The listing builds one solid part. Answer for the finished solid, in the listing's coordinates (mm). Give positions to 0.01 mm unless a question says otherwise; leave off trailing zeros. Write each loop counter-clockwise with the first axis right and the second up, starting at its lowest first coordinate (ties: lowest second). Pieces come first, ordered by that corner, then holes. Notation, with made-up numbers: (84, -2.75) -> (88, -2.75) arc R19 ccw to (88, 9.25) -> close; hole circle Ø7 at (74.5, 89.25). An arc over 180 degrees is marked (long way). One line per question, with ' | ' between items.
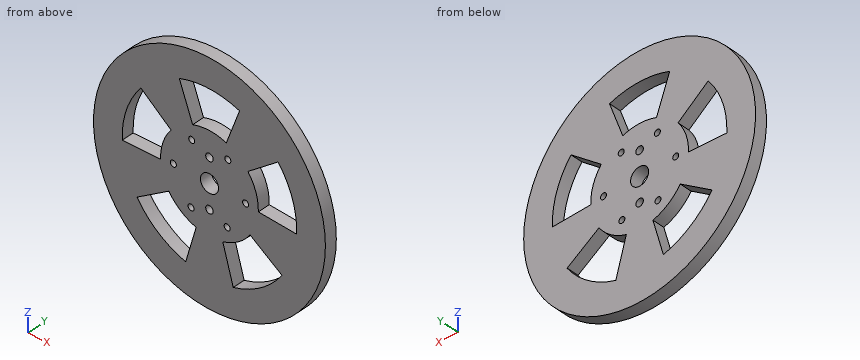
from build123d import *

# Parameters (mm, degrees)
F0_R            = 244.475
F0_R_2          = 6.35
F0_R_3          = 7.9375
F0_R_4          = 19.05
F1_DEPTH        = 25.4
F3_DEPTH        = 25.4
F3_COPIES_COUNT = 5


# Not quite as in the source:
# - a pattern or mirror of a feature is missing from the dataset's text; its kind, count and spacing are read off the source's solid


with BuildPart() as f1:
    # F0 (on Front) → F1 (new body)
    with BuildSketch(Plane.XZ):
        Circle(F0_R)
        with Locations((-38.7905028095, -65.5876275817)):
            Circle(F0_R_2, mode=Mode.SUBTRACT)
        with Locations((37.4053002549, -66.3873746494)):
            Circle(F0_R_2, mode=Mode.SUBTRACT)
        with Locations((0, -50.8)):
            Circle(F0_R_3, mode=Mode.SUBTRACT)
        with Locations((76.1958030644, -0.7997470677)):
            Circle(F0_R_2, mode=Mode.SUBTRACT)
        with Locations((-76.1958030644, 0.7997470677)):
            Circle(F0_R_2, mode=Mode.SUBTRACT)
        with Locations((-37.4053002549, 66.3873746494)):
            Circle(F0_R_2, mode=Mode.SUBTRACT)
        Circle(F0_R_4, mode=Mode.SUBTRACT)
        with Locations((0, 50.8)):
            Circle(F0_R_3, mode=Mode.SUBTRACT)
        with Locations((38.7905028095, 65.5876275817)):
            Circle(F0_R_2, mode=Mode.SUBTRACT)
    extrude(amount=F1_DEPTH)

    # F2 (on Front) → F3 (cut, through all)
    with BuildSketch(Plane.XZ):
        with BuildLine():
            ThreePointArc((-35.5586123208, 96.7233082276), (0, 103.0524782073), (35.5586123208, 96.7233082276))
            Line((35.5586123208, 96.7233082276), (63.5, 172.7269336903))
            ThreePointArc((63.5, 172.7269336903), (0, 184.0294640053), (-63.5, 172.7269336903))
            Line((-63.5, 172.7269336903), (-35.5586123208, 96.7233082276))
        make_face()
    f3 = extrude(amount=F3_DEPTH, mode=Mode.SUBTRACT)

    # F3_copies: F3 ×5 about axis
    f3_copies_axis = Axis((0, 0, 0), (0, 1, 0))
    for i in range(1, F3_COPIES_COUNT):
        add(f3.rotate(f3_copies_axis, i * 360 / F3_COPIES_COUNT), mode=Mode.SUBTRACT)


solid = f1.part
Item 1: Find section A-A (x = 0). Count the separate pieces of the cut face and the enclosed holes in it, then the cut area to 3 significant figures.
Answers below:
separate pieces: 5 | enclosed holes: 0 | area: 8,590 mm²
Item 2: Find section D-D (z = 50.8). Write down the section's boundary in (x, y).
Answers below:
outline: (-239.14, -25.4) -> (-176.88, -25.4) -> (-176.88, 0) -> (-239.14, 0) -> close; (-89.66, -25.4) -> (-7.94, -25.4) -> (-7.94, 0) -> (-89.66, 0) -> close; (7.94, -25.4) -> (89.66, -25.4) -> (89.66, 0) -> (7.94, 0) -> close; (176.88, -25.4) -> (239.14, -25.4) -> (239.14, 0) -> (176.88, 0) -> close
Item 3: Find section B-B (z = -156.5). Write down the section's boundary in (x, y), then the cut area to 3 significant figures.
Answers below:
outline: (-187.82, -25.4) -> (-96.82, -25.4) -> (-96.82, 0) -> (-187.82, 0) -> close; (-44.33, -25.4) -> (44.33, -25.4) -> (44.33, 0) -> (-44.33, 0) -> close; (96.82, -25.4) -> (187.82, -25.4) -> (187.82, 0) -> (96.82, 0) -> close | area: 6,870 mm²
Item 4: Find section C-C (x = 127.5). Write down the section's boundary in (y, z).
Answers below:
outline: (-25.4, -208.59) -> (0, -208.59) -> (0, -132.7) -> (-25.4, -132.7) -> close; (-25.4, -85.4) -> (0, -85.4) -> (0, -4.86) -> (-25.4, -4.86) -> close; (-25.4, 100.28) -> (0, 100.28) -> (0, 208.59) -> (-25.4, 208.59) -> close
Item 5: Flat-ended cylindrical pins translate along their axes: pin 1 (6 mm diameter, centred on y = -21, z = 150, fed in from +X); pin 2 (2 mm diameter, centred on y = -17, z = 23.5, fed in from -X); pin 3 (3 mm diameter, centred on x = -154.5, y = -17, fed in from -Z). Find the tip coordinate at first contact, or state that the pin passes through.
Answers below:
pin 1: x = 195.34 | pin 2: x = -243.44 | pin 3: z = -190.68
Item 6: Consider line 1 (Z direction, x = 92.5, y = -7.5); line 2 (X direction, y = -10.75, z = 63); line 3 (X direction, y = -7, z = 92). Determine where each line is inside the solid, lowest interval first. Write a range as [from, to].
Answers below:
line 1: [-226.3, -159.09], [-61.96, 45.43], [72.75, 226.3] | line 2: [-236.22, -172.91], [-81.55, -42.78], [-32.03, 32.99], [44.59, 81.55], [172.91, 236.22] | line 3: [-226.5, -159.38], [-116.97, 116.97], [159.38, 226.5]
